Verification items for this drawing (mm, ordinates from the low corner). A direction names the side the tool comes from. Coordinates: 2 decimals unless noted, no trailing zeros. Order: outer loops, then holes, each group sorted by start corner. A loop starts at its lowest first (then second) coordinate and runs counter-clockwise, first axis right, second up. Notation, with made-up numbers: M -20.5,15.5 L -12.5,15.5 A26 cw -12.5,40.5 Z; hole C -2,34.5 d7. An arc over 180 degrees is marked long. Answer as a JSON object with one key per item and string values. Group by question number.
(1) Gauge pin test, flat ends, axial feed: pin 1 Ø15 at (x, z) = (38.56, 24.61) entering from +Y; pin 2 Ø5 at (x, y) = (18, 83) entering from -Z; pin 3 Ø3 at (x, y) = (2.5, 45) entering from +Z; pin 4 Ø6 at (x, y) = (52.5, 33.5) entering from +Z. Record the tip position at first contact, or that the pin passes through.
(2) Cross-section at A-A (z = 40.5). Enter the section's corners in (x, y) (1 decimal).
(3) Material ranges on line 1 (Y direction, x = 44.5, z = 45.5) (1 decimal); line 2 (X direction, y = 66, z = 15.5) (1 decimal); line 3 (Z direction, x = 66.5, y = 32), recorded low to high.
(4) Access from +Z, -Z, +X, -X, +Y, -Y to the whole of each face (thin tool, end or side, straight path). Record for the marked faces 1 and 2.
(5) Mould release check, pull along X, two halves, no side actions. Record for the marked faces 3, 4 and 5: released by +X, released by -X, zero draft, split by the parting line, or undercut.
(6) Cross-section at B-B (x = 52). Enter the section's corners in (y, z) (1 decimal).
(7) Cross-section at C-C (y = 57.5). Enter the section's corners in (x, z) (1 decimal).
(8) Cross-section at D-D (z = 30.5). Enter the section's corners in (x, y) (1 decimal).
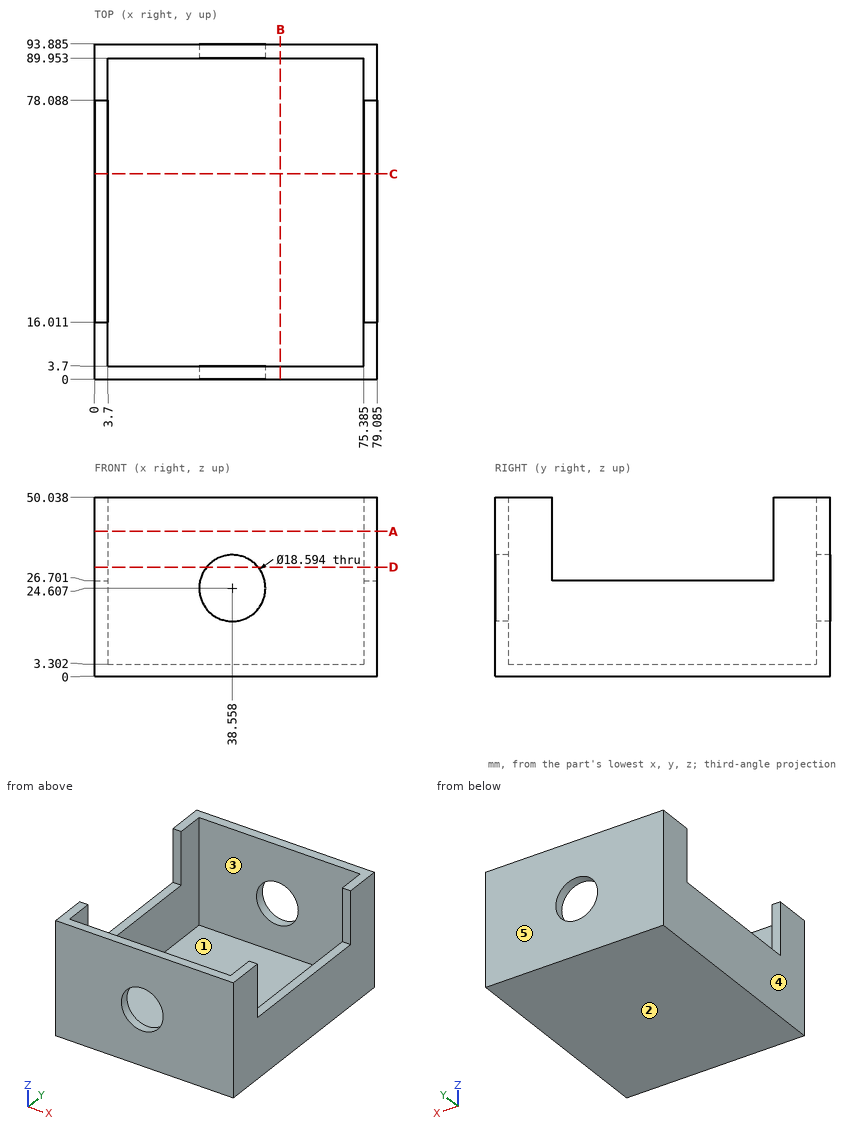
Taken from the geometry:
{
 "1": {"pin 1": "passes through", "pin 2": "stops at z = 0", "pin 3": "stops at z = 26.7", "pin 4": "stops at z = 3.3"},
 "2": {"outline": "M 0,0 L 79.1,0 L 79.1,16 L 75.4,16 L 75.4,3.7 L 3.7,3.7 L 3.7,16 L 0,16 Z; M 0,78.1 L 3.7,78.1 L 3.7,90 L 75.4,90 L 75.4,78.1 L 79.1,78.1 L 79.1,93.9 L 0,93.9 Z"},
 "3": {"line 1": "y = 0 to 3.7, 90 to 93.9", "line 2": "x = 0 to 3.7, 75.4 to 79.1", "line 3": "z = 0 to 3.3"},
 "4": {"face 1": "+Z", "face 2": "-Z, +X, -X, +Y, -Y"},
 "5": {"face 3": "undercut", "face 4": "released by -X", "face 5": "zero draft"},
 "6": {"outline": "M 0,0 L 93.9,0 L 93.9,50 L 90,50 L 90,3.3 L 3.7,3.3 L 3.7,50 L 0,50 Z"},
 "7": {"outline": "M 0,0 L 79.1,0 L 79.1,26.7 L 75.4,26.7 L 75.4,3.3 L 3.7,3.3 L 3.7,26.7 L 0,26.7 Z"},
 "8": {"outline": "M 0,0 L 31.4,0 L 31.4,3.7 L 3.7,3.7 L 3.7,16 L 0,16 Z; M 0,78.1 L 3.7,78.1 L 3.7,90 L 31.4,90 L 31.4,93.9 L 0,93.9 Z; M 45.7,0 L 79.1,0 L 79.1,16 L 75.4,16 L 75.4,3.7 L 45.7,3.7 Z; M 45.7,90 L 75.4,90 L 75.4,78.1 L 79.1,78.1 L 79.1,93.9 L 45.7,93.9 Z"}
}
